Part model, mm, in its own coordinate system. Face numbers are marked on the shaded views. A direction names the side the tool comes from. Give positions to 0.01 mm unless a question says otherwise; leave off trailing zeros. Order: outer loops, then holes, each group sorted by start corner. A loop starts at its lowest first (then second) coordinate and runs counter-clockwise, first axis right, second up. Notation, with made-up numbers: (80.25, -25.5) -> (94.25, -25.5) arc R21 cw to (94.25, -18.5) -> close; hole circle Ø11 at (59, 16.25). An arc over 180 degrees is marked (long way). Write item = value, one per line. Start each with the question number.
Item 1: Band-saw the part on A-A on y = -57.5. Write the cut outline in (x, z), plus the area to 3 significant figures.
Item 2: Pull direction Y, two halves, no side cores. Call the marked faces 1, 2 and 3: +Y half, -Y half, draft (parallel to the pull), parting line (faces both ways), or undercut.
Item 3: Band-saw the part on B-B on x = 119. Write the cut outline in (y, z), plus the area to 3 significant figures.
Item 4: Flat gauge pins, fed straight in: P1, Ø8, axis at x = 243.5, y = -41.5, coming from the +Z side; P2, Ø2, axis at x = 357.5, y = -39.5, coming from the -Z side. Where does each tip first touch, or does it go through?
Item 5: Tool access for the marked faces 4 and 5: list every direction of +Z, -Z, +X, -X, +Y, -Y with a clear straight run to the whole face (end or side of a thin tool).
Item 6: Drill centre lines: line 1 along X through (y, z) = (120, 118); line 2 along Y through (x, z) = (90, 146); line 3 along Z through (x, y) = (113.5, -32). Where is each one in solid material? Low to high.
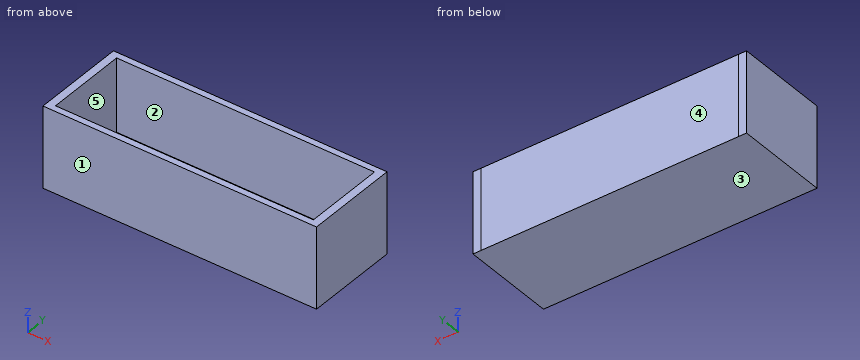
```python
from build123d import *

# Parameters (mm, degrees)
F0_W     = 825
F0_H     = 20
F1_DEPTH = 260
F0_H_2   = 260
F2_DEPTH = 25


# Not quite as in the source:
# - ends of sketch curves that miss each other by under 0.0002 mm in the source are joined
# - a feature names something its author has since deleted; it is built from what else it names


with BuildPart() as f1:
    # F0 (on Top) → F1 (new body)
    with BuildSketch(Plane.XY):
        Polygon((422.5, 130), (422.5, 149.9999940395), (-402.5, 150), (-402.5, 130), align=None)
        Polygon((422.5, -150), (447.5, -150), (447.5, 150), (422.5, 150), (422.5, 130), (422.5, -130), align=None)
        with Locations((10, -140)):
            Rectangle(F0_W, F0_H)
        Polygon((-427.5, -150), (-402.5, -150), (-402.5, -130), (-402.5, 130), (-402.5, 149.9999940395), (-427.5, 150), align=None)
    extrude(amount=F1_DEPTH)

    # F0 (on Top) → F2 (join)
    with BuildSketch(Plane.XY):
        with Locations((10, 0)):
            Rectangle(F0_W, F0_H_2)
    extrude(amount=F2_DEPTH)


solid = f1.part
```
Values found:
q1.outline = (-427.5, 0) -> (447.5, 0) -> (447.5, 260) -> (422.5, 260) -> (422.5, 25) -> (-402.5, 25) -> (-402.5, 260) -> (-427.5, 260) -> close
q1.area = 33,600 mm^2
q2.face_1 = -Y half
q2.face_2 = undercut
q2.face_3 = draft
q3.outline = (-150, 0) -> (150, 0) -> (150, 260) -> (130, 260) -> (130, 25) -> (-130, 25) -> (-130, 260) -> (-150, 260) -> close
q3.area = 16,900 mm^2
q4.P1 = 25
q4.P2 = 0
q5.face_4 = +Z, -Z, +X, -X, +Y
q5.face_5 = +Z
q6.line_1 = -427.5 to -402.5, 422.5 to 447.5
q6.line_2 = -150 to -130, 130 to 150
q6.line_3 = 0 to 25
